Source: CAD feature listing. Evaluate the final solid. Frame: model axes, mm. A direction names the side the tool comes from. Give positions to 0.01 mm unless a question says otherwise; leave off trailing zeros. Order: outer loops, then holes, each group sorted by start corner. A loop starts at its lowest first (then second) coordinate and runs counter-clockwise, first axis right, second up. Notation, with made-up numbers: M 0.5,66.5 L 54.5,66.5 A19 ccw 54.5,87.5 Z; hole C 59.25,-37.75 d7. An arc over 180 degrees is marked long. Answer in a Markdown table with one row per item. Add a question column.
(1) Set-up query: faces 3 (the face through (0, 0, 30)), 4 (the face through (-0.867, -3.905, -3.028)). Return all of +Z, -Z, +X, -X, +Y, -Y with unobstructed straight access to the full face (end or side cutting, diameter ignored); none if empty.
(2) Section query D-D, the plane z = -12.5. Return loops of the section in (x, y).
(3) Section query A-A, the plane x = 0. Return loops of the section in (y, z), plus the area to 3 significant figures.
(4) Section query C-C, the plane z = 25. Return loops of the section in (x, y), plus the area to 3 significant figures.
(5) Mould query, pull axis Z, two halves, no side actions, for faces 1 (the face through (6.466, -2.681, -11.056)), 2 (the face through (-1, -2, 0)). Classes: pulls with the +Z half, pulls with the -Z half, needs draft (parallel to the pull), parting line crosses it, or undercut.
(6) Material intervals for line 1 along X through (y, z) = (0.25, -13); line 2 along Z through (x, y) = (0.25, -1.5); line 3 along Y through (x, z) = (-3.5, -13), sorted ascending.
(7) Pin query (flat end, axial travel): P1, Ø6, axis at y = -4, z = -10, coming from the +X side; P2, Ø4, axis at x = 5, y = -4.5, coming from the -Z side; P3, Ø1.5, axis at y = -3, z = -2.5, coming from the +X side; P4, Ø1, axis at x = -3, z = 10, coming from the +Y side. Return the tip coordinate at first contact, or that it passes through.
from build123d import *

# Parameters (mm, degrees)
SKETCH2_R           = 2
BOSS_EXTRUDE1_DEPTH = 30
FILLET1_R           = 2
FILLET2_R           = 1


with BuildPart() as part:
    # Sketch1 → Revolve1 (revolve)
    with BuildSketch(Plane(origin=(0, 0, 0), x_dir=(1, 0, 0), z_dir=(0, 1, 0))):
        with BuildLine():
            Line((0, 0), (4, 0))
            Line((4, 0), (4, 5))
            Line((4, 5), (7, 5))
            Line((7, 5), (7, 15))
            Line((7, 15), (6.5, 15))
            ThreePointArc((6.5, 15), (4.596194078, 19.596194078), (0, 21.5))
            Line((0, 21.5), (0, 0))
        make_face()
    revolve(axis=Axis((0, 0, -21.5), (0, 0, 1)))

    # Sketch2 → Boss-Extrude1 (add)
    with BuildSketch(Plane.XY):
        Circle(SKETCH2_R)
    extrude(amount=BOSS_EXTRUDE1_DEPTH)

    # Fillet1
    fillet1_edges = [part.edges().sort_by_distance(p)[0] for p in [
        (-7, 0, -5),
    ]]
    fillet(fillet1_edges, radius=FILLET1_R)

    # Fillet2
    fillet2_edges = [part.edges().sort_by_distance(p)[0] for p in [
        (-4, 0, 0),
    ]]
    fillet(fillet2_edges, radius=FILLET2_R)


solid = part.part
Values follow:
| question | item | result |
|---|---|---|
| 1 | face 3 | +Z, +X, -X, +Y, -Y |
| 1 | face 4 | +Z |
| 2 | outline | C 0,0 d14 |
| 3 | outline | M -7,-15 L -6.5,-15 A6.5 ccw 6.5,-15 L 7,-15 L 7,-7 A2 ccw 5,-5 L 4,-5 L 4,-1 A1 ccw 3,0 L 2,0 L 2,30 L -2,30 L -2,0 L -3,0 A1 ccw -4,-1 L -4,-5 L -5,-5 A2 ccw -7,-7 Z |
| 3 | area | 364 mm² |
| 4 | outline | C 0,0 d4 |
| 4 | area | 12.6 mm² |
| 5 | face 1 | needs draft |
| 5 | face 2 | pulls with the +Z half |
| 6 | line 1 | x = -7 to 7 |
| 6 | line 2 | z = -21.32 to 30 |
| 6 | line 3 | y = -6.06 to 6.06 |
| 7 | P1 | stops at x = 6.93 |
| 7 | P2 | stops at z = -19.46 |
| 7 | P3 | stops at x = 3.31 |
| 7 | P4 | passes through |
